```python
from build123d import *

# Parameters (mm, degrees)
PAD_DEPTH       = 54
SKETCH001_R     = 1.6
POCKET_DEPTH    = 6
SKETCH002_R     = 6.1
POCKET001_DEPTH = 5


with BuildPart() as part:
    # Sketch → Pad (new body)
    with BuildSketch(Plane.XY):
        Polygon((0, 0), (0, 6), (9, 6), (9, 40), (53, 40), (53, 6), (62, 6), (62, 0), (49, 0), (49, 36), (13, 36), (13, 0), align=None)
    extrude(amount=PAD_DEPTH)

    # Sketch001 (on Face8 of Pad) → Pocket (cut)
    with BuildSketch(Plane.XZ):
        with Locations((5, 5)):
            Circle(SKETCH001_R)
        with Locations((57, 5)):
            Circle(SKETCH001_R)
        with Locations((57, 49)):
            Circle(SKETCH001_R)
        with Locations((5, 49)):
            Circle(SKETCH001_R)
    extrude(amount=-POCKET_DEPTH, mode=Mode.SUBTRACT)

    # Sketch002 (on Face10 of Pocket) → Pocket001 (cut)
    with BuildSketch(Plane(origin=(0, 40, 0), x_dir=(-1, 0, 0), z_dir=(0, 1, 0))):
        with Locations((-31, 26)):
            Circle(SKETCH002_R)
    extrude(amount=-POCKET001_DEPTH, mode=Mode.SUBTRACT)


solid = part.part
```
Build history of the part. All positions in model axes, mm. A direction names the side the tool comes from. Round coordinates to 2 decimals unless told otherwise and drop trailing zeros. Write each loop counter-clockwise with the first axis right and the second up, starting at its lowest first coordinate (ties: lowest second). Pieces come first, ordered by that corner, then holes.
1) Band-saw the part on C-C, the plane x = 5. List the corners of the cut face in (y, z), and give its area (3 significant figures).
2) Band-saw the part on A-A, the plane y = 8.5. List the corners of the cut face in (x, z).
3) Band-saw the part on D-D, the plane z = 21. List the corners of the cut face in (x, y).
4) Mould opens along X. For faces 1 (the flat face through (0, 3, 27)), 2 (the flat face through (31, 36, 33)), 3 (the flat face through (33.4, 36.4, 0)) say: +X half, -X half, draft (parallel to the pull), parting line (faces both ways), or undercut.
5) 3-axis set-ups, long thin cutter, end or side, ignore diameter. For faces 4 (the flat face through (7, 0, 27)), 5 (the flat face through (4, 6, 27)), 6 (the flat face through (57, 6, 27)), 7 (the flat face through (13, 18, 27)): which of +Z, -Z, +X, -X, +Y, -Y reach the whole face in a straight line?
6) Band-saw the part on B-B, the plane z = 5. List the corners of the cut face in (x, y).
7) Pin check, flat tips, straight feed: pin 1 (1 mm diameter, centred on y = 8.5, z = 24.5, fed in from +X); pin 2 (11 mm diameter, centred on y = 18, z = 22, fed in from -X); pin 3 (16 mm diameter, centred on x = 31, z = 26, fed in from +Y); pin 4 (4.5 mm diameter, centred on x = 3, z = 28.5, fed in from +Y). Stop position of each tip, or through.
8) Drill centre lines: probe 1 along Z at (x, y) = (5, 1); probe 2 along X at (y, z) = (6.5, 21); probe 3 along X at (y, z) = (2.5, 33.5). Where is each one in solid material? Low to high.
Ans:
1. outline: (0, 0) - (6, 0) - (6, 3.4) - (0, 3.4) - close; (0, 6.6) - (6, 6.6) - (6, 47.4) - (0, 47.4) - close; (0, 50.6) - (6, 50.6) - (6, 54) - (0, 54) - close
1. area: 286 mm2
2. outline: (9, 0) - (13, 0) - (13, 54) - (9, 54) - close; (49, 0) - (53, 0) - (53, 54) - (49, 54) - close
3. outline: (0, 0) - (13, 0) - (13, 36) - (27.51, 36) - (27.51, 40) - (9, 40) - (9, 6) - (0, 6) - close; (34.49, 36) - (49, 36) - (49, 0) - (62, 0) - (62, 6) - (53, 6) - (53, 40) - (34.49, 40) - close
4. face 1: -X half
4. face 2: undercut
4. face 3: draft
5. face 4: +Z, -Z, +X, -X, -Y
5. face 5: +Z, -Z, -X, +Y
5. face 6: +Z, -Z, +X, +Y
5. face 7: +Z, -Z, -Y
6. outline: (0, 0) - (3.4, 0) - (3.4, 6) - (0, 6) - close; (6.6, 0) - (13, 0) - (13, 36) - (49, 36) - (49, 0) - (55.4, 0) - (55.4, 6) - (53, 6) - (53, 40) - (9, 40) - (9, 6) - (6.6, 6) - close; (58.6, 0) - (62, 0) - (62, 6) - (58.6, 6) - close
7. pin 1: stops at x = 53
7. pin 2: stops at x = 9
7. pin 3: stops at y = 40
7. pin 4: stops at y = 6
8. probe 1: z = 0 to 3.4, 6.6 to 47.4, 50.6 to 54
8. probe 2: x = 9 to 13, 49 to 53
8. probe 3: x = 0 to 13, 49 to 62
